Verification items for the finished model (mm, model axes). A direction names the side the tool comes from. Coordinates: 2 decimals unless noted, no trailing zeros. Order: outer loops, then holes, each group sorted by start corner. A loop starts at its lowest first (then second) coordinate and runs counter-clockwise, first axis right, second up. Notation, with made-up numbers: M -7,86 L 49,86 A26 cw 49,112 Z; hole C 25.5,10.25 d3. An arc over 180 degrees is marked long. Answer as a JSON object with one key per item and string values. Group by question number.
(1) Access from +Z, -Z, +X, -X, +Y, -Y to the whole of each face (thin tool, end or side, straight path). Record for faces 1 (the face through (-3, 17.1, -9.54)), 2 (the face through (-14.3, 25.5, -3.6)), 3 (the face through (15.62, 23.98, 3.47)).
(2) Cross-section at A-A (y = 16). Enter the section's corners in (x, z).
(3) Cross-section at C-C (x = 0). Count the separate pieces of the cut face and the enclosed holes in it, plus the area to 3 significant figures.
(4) Material ranges on line 1 (Y direction, x = -12.5, z = -8); line 2 (X direction, y = 15, z = 0); line 3 (Y direction, x = 11, z = -11.5), recorded low to high.
(5) Cross-section at D-D (y = 28). Enter the section's corners in (x, z).
(6) Gauge pin test, flat ends, axial feed: pin 1 Ø4 at (x, y) = (0, 16) entering from -Z; pin 2 Ø13 at (x, z) = (-4.5, 4.5) entering from -Y; pin 3 Ø1 at (x, z) = (-12, 1.5) entering from +Y; pin 4 Ø9.5 at (x, z) = (-7, 5.5) entering from +Y. Record the tip position at first contact, or that the pin passes through.
(7) Mould release check, pull along Z, two halves, no side actions. Record for faces 4 (the face through (0, 24, 0)), 5 (the face through (4.155, 31.585, 0.923)), 6 (the face through (-13.1, 0, 1.3)): released by +Z, released by -Z, zero draft, split by the parting line, or undercut.
from build123d import *

# Parameters (mm, degrees)
CUT_EXTRUDE1_DEPTH      = 39
CUT_EXTRUDE1_DEPTH_BACK = 50
SKETCH2_R               = 2.5


with BuildPart() as part:
    # Sketch1 → Revolve2 (revolve)
    with BuildSketch(Plane.XY, mode=Mode.PRIVATE) as revolve2_sk:
        with BuildLine():
            Line((13, 0), (13, 10))
            Line((13, 10), (10, 10))
            Line((10, 10), (10, 24))
            Line((10, 24), (0, 24))
            Line((0, 24), (0, 32))
            Line((0, 32), (0, 32.027132664))
            ThreePointArc((0, 32.027132664), (1.743114855, 31.951026626), (3.472963553, 31.723287724))
            Line((3.472963553, 31.723287724), (16, 29.51443321))
            Line((16, 29.51443321), (16, 27))
            Line((16, 27), (14.5, 27))
            Line((14.5, 27), (14.5, 25.5))
            Line((14.5, 25.5), (16, 25.5))
            Line((16, 25.5), (16, 22.5))
            Line((16, 22.5), (14.5, 22.5))
            Line((14.5, 22.5), (14.5, 21))
            Line((14.5, 21), (16, 21))
            Line((16, 21), (16, 0))
            Line((16, 0), (13, 0))
        make_face()
    revolve(revolve2_sk.sketch.rotate(Axis((0, 0, 0), (0, 1, 0)), 90), axis=Axis((0, 0, 0), (0, 1, 0)))

    # Sketch2 → Cut-Extrude1 (cut, two sides: drawn at the far end of the back side and taken through both)
    with BuildSketch(Plane.XY.offset(-CUT_EXTRUDE1_DEPTH_BACK)):
        with Locations(Location((0, 16, 0), (0, 0, 180))):
            Circle(SKETCH2_R)
    extrude(amount=CUT_EXTRUDE1_DEPTH + CUT_EXTRUDE1_DEPTH_BACK, mode=Mode.SUBTRACT)


solid = part.part
Taken from the geometry:
{
 "1": {"face 1": "-Y", "face 2": "none", "face 3": "+Y, -Y"},
 "2": {"outline": "M -2.5,-15.8 L -2.5,-9.68 A10 cw -2.5,9.68 L -2.5,15.8 A16 ccw Z; M 2.5,-15.8 A16 ccw 2.5,15.8 L 2.5,9.68 A10 cw 2.5,-9.68 Z"},
 "3": {"separate pieces": "3", "enclosed holes": "0", "area": "380 mm²"},
 "4": {"line 1": "y = 0 to 21, 22.5 to 25.5, 27 to 29.72", "line 2": "x = -16 to -10, 10 to 16", "line 3": "y = 0 to 21, 22.5 to 25.5, 27 to 29.53"},
 "5": {"outline": "C 0,0 d32"},
 "6": {"pin 1": "passes through", "pin 2": "stops at y = 10", "pin 3": "stops at y = 30.29", "pin 4": "stops at y = 31.6"},
 "7": {"face 4": "undercut", "face 5": "split by the parting line", "face 6": "zero draft"}
}
